Here's how the part is built. I have some questions about the finished solid (model axes, mm). Round coordinates to 2 decimals unless told otherwise and drop trailing zeros. Write each loop counter-clockwise with the first axis right and the second up, starting at its lowest first coordinate (ties: lowest second). Pieces come first, ordered by that corner, then holes. Notation, with made-up numbers: (-16.75, -10) -> (-6.75, -10) arc R12 ccw to (-6.75, 0) -> close; hole circle Ø6 at (-39, 30). An arc over 180 degrees is marked (long way). Put each result on its own line as item: value. Start each with the question number.
1. Suppose I cut it at C-C (z = 8). Please give me the cut outline in (x, y), then the cut area to 3 significant figures.
2. I need wall thicknesses on probe 1 along Y at (x, z) = (1, 3.75); probe 2 along X at (y, z) = (0.5, 2.75); probe 3 along Z at (x, y) = (-23, -30). Which ranges of each line are inside material? Lowest first, please. Write a range as from..to.
3. We'd pull the mould along X, two halves only. Please class faces 1 (the face through (40.06, 12.62, 5.93)), 2 (the face through (37.1, -15.4, 11)), 3 (the face through (-33, 15, 3)), 4 (the face through (-8.67, -39.05, 6.94)): +X half, -X half, draft (parallel to the pull), parting line (faces both ways), or undercut.
4. For pin 1 (2 mm diameter, centred on x = 24.5, z = 3, fed in from +Y); pin 2 (6 mm diameter, centred on x = 16, z = 8.5, fed in from -Y); pin 3 (2 mm diameter, centred on x = -8.5, z = 3.5, fed in from +Y), each with a flat end and sliding along its axis, tell me the tip position at first contact or that it passes through.
5. Suppose I cut it at A-A (y = 0). Please give me the cut outline in (x, z), then the cut area to 3 significant figures.
```python
from build123d import *

# Parameters (mm, degrees)
F0_R     = 40
F0_R_2   = 36
F1_DEPTH = 3
F0_R_3   = 42
F2_DEPTH = 11
F3_R     = 1
F4_R     = 1


with BuildPart() as f1:
    # F0 (on Top) → F1 (new body)
    with BuildSketch(Plane.XY):
        Circle(F0_R)
        Circle(F0_R_2, mode=Mode.SUBTRACT)
    extrude(amount=F1_DEPTH)

    # F0 (on Top) → F2 (join)
    with BuildSketch(Plane.XY):
        Circle(F0_R_3)
        Circle(F0_R, mode=Mode.SUBTRACT)
    extrude(amount=F2_DEPTH)

    # F3
    f3_edges = [f1.edges().sort_by_distance(p)[0] for p in [
        (-42, 0, 0),
    ]]
    fillet(f3_edges, radius=F3_R)

    # F4
    f4_edges = [f1.edges().sort_by_distance(p)[0] for p in [
        (-36, 0, 0),
    ]]
    fillet(f4_edges, radius=F4_R)


solid = f1.part
```
Verdict:
1. outline: circle Ø84 at (0, 0); hole circle Ø80 at (0, 0)
1. area: 515 mm^2
2. probe 1: y = -41.99..-39.99, 39.99..41.99
2. probe 2: x = -42..-36, 36..42
2. probe 3: z = 0..3
3. face 1: parting line
3. face 2: draft
3. face 3: undercut
3. face 4: undercut
4. pin 1: stops at y = 34.81
4. pin 2: stops at y = -39.94
4. pin 3: stops at y = 41.32
5. outline: (-42, 1) arc R1 ccw to (-41, 0) -> (-37, 0) arc R1 ccw to (-36, 1) -> (-36, 3) -> (-40, 3) -> (-40, 11) -> (-42, 11) -> close; (36, 1) arc R1 ccw to (37, 0) -> (41, 0) arc R1 ccw to (42, 1) -> (42, 11) -> (40, 11) -> (40, 3) -> (36, 3) -> close
5. area: 67.1 mm^2
